from build123d import *

# Parameters (mm, degrees)
CUT_EXTRUDE1_DEPTH = 4
CHAMFER1_SIZE      = 0.5
CHAMFER2_SIZE      = 0.5


with BuildPart() as part:
    # Sketch1 → Revolve1 (revolve)
    with BuildSketch(Plane.XY, mode=Mode.PRIVATE) as revolve1_sk:
        Polygon((0, 11.5), (4.5, 11.5), (4.5, 6.5), (2.5, 6.5), (2.5, -11.5), (0, -11.5), align=None)
    revolve(revolve1_sk.sketch.rotate(Axis((0, 14.918478261, 0), (0, -1, 0)), 90), axis=Axis((0, 14.918478261, 0), (0, -1, 0)))

    # Sketch2 → Cut-Extrude1 (cut)
    with BuildSketch(Plane(origin=(0, 11.5, 0), x_dir=(1, 0, 0), z_dir=(0, 1, 0))):
        Polygon((0, 2.309401077), (-2, 1.154700538), (-2, -1.154700538), (0, -2.309401077), (2, -1.154700538), (2, 1.154700538), align=None)
    extrude(amount=-CUT_EXTRUDE1_DEPTH, mode=Mode.SUBTRACT)

    # Chamfer1
    chamfer1_edges = [part.edges().sort_by_distance(p)[0] for p in [
        (0, 11.5, -4.5),
    ]]
    chamfer(chamfer1_edges, length=CHAMFER1_SIZE)

    # Chamfer2
    chamfer2_edges = [part.edges().sort_by_distance(p)[0] for p in [
        (0, -11.5, -2.5),
    ]]
    chamfer(chamfer2_edges, length=CHAMFER2_SIZE)


solid = part.part
Here's how the part is built. I have some questions about the finished solid (model axes, mm). A direction names the side the tool comes from. Give positions to 0.01 mm unless a question says otherwise; leave off trailing zeros. Order: outer loops, then holes, each group sorted by start corner. A loop starts at its lowest first (then second) coordinate and runs counter-clockwise, first axis right, second up. Notation, with made-up numbers: M -28,14 L 29,14 A36 cw 29,48 Z; hole C 82,75 d7. An arc over 180 degrees is marked long. Answer as a JSON object with one key per item and string values. Group by question number.
1) Suppose I cut it at B-B, the plane y = -1.5. Write out the boundary of the cut face in (x, z), plus the area to 3 significant figures.
2) I'm going to push flat-ended pins straight in: pin 1 Ø2 at (y, z) = (-3.5, 0) entering from +X; pin 2 Ø4 at (y, z) = (-0.5, 3) entering from +X; pin 3 Ø2 at (y, z) = (1.5, 2.5) entering from -X. Where does each tip first touch, or does it pass through?
3) Suppose I cut it at A-A, the plane z = 0. Write out the boundary of the cut face in (x, y).
4) On a 3-axis mill with a long thin cutter (end or side, diameter ignored), from which of +Z, -Z, +X, -X, +Y, -Y can I reach the whole of each face in a straight line? I mean faces 1 (the flat face through (1, 11.5, 2)), 2 (the flat face through (1.014, 9.528, -1.724)). Say none if no direction works.
5) Please list where these lines run through material, in increasing order: L1, parallel to Y at x = 0.5, z = 3.25; L2, parallel to X at y = -4, z = -1.5; L3, parallel to X at y = 9.5, z = -1.25. Write a range as [from, to].
6) We'd pull the mould along Z, two halves only. Please class faces 3 (the flat face through (2, 10, 0)), 4 (the cylindrical face through (-0.1, -2.4, -2.5)), 5 (the flat face through (2, 6.5, 2)): pulls with the +Z half, pulls with the -Z half, needs draft (parallel to the pull), parting line crosses it, or undercut.
Results found:
{
 "1": {"outline": "C 0,0 d5", "area": "19.6 mm²"},
 "2": {"pin 1": "x = 2.5", "pin 2": "x = 2.29", "pin 3": "x = -2"},
 "3": {"outline": "M -4.5,6.5 L -2.5,6.5 L -2.5,-11 L -2,-11.5 L 2,-11.5 L 2.5,-11 L 2.5,6.5 L 4.5,6.5 L 4.5,11 L 4,11.5 L 2,11.5 L 2,7.5 L -2,7.5 L -2,11.5 L -4,11.5 L -4.5,11 Z"},
 "4": {"face 1": "+Z, -Z, +X, -X, +Y", "face 2": "+Y"},
 "5": {"L1": "[6.5, 11.5]", "L2": "[-2, 2]", "L3": "[-4.32, -1.83], [1.83, 4.32]"},
 "6": {"face 3": "undercut", "face 4": "parting line crosses it", "face 5": "needs draft"}
}
